```python
from build123d import *

# Parameters (mm, degrees)
BOSS_EXTRUDE1_DEPTH   = 25.4
FILLET1_R             = 6.35
F_8_CLEARANCE_HOLE1_D = 4.4958
F_8_CLEARANCE_HOLE2_D = 4.4958


with BuildPart() as part:
    # Sketch1 → Boss-Extrude1 (new body)
    with BuildSketch(Plane(origin=(0, 0, 0), x_dir=(0, 0, -1), z_dir=(1, 0, 0))):
        Polygon((0, 0), (0, 38.1), (-3.175, 38.1), (-3.175, 3.175), (-38.1, 3.175), (-38.1, 0), align=None)
    extrude(amount=BOSS_EXTRUDE1_DEPTH)

    # Fillet1
    # the kernel refuses this fillet: 6.35 mm, written as the material it adds along each edge
    with BuildSketch(Plane(origin=(0, 3.175, 3.175), x_dir=(0, 1, 0), z_dir=(1, 0, 0))) as fillet1_piece_1:
        with BuildLine():
            CenterArc((FILLET1_R, FILLET1_R), FILLET1_R, 180, 90)
            Line((0, FILLET1_R), (0, 0))
            Line((0, 0), (FILLET1_R, 0))
        make_face()
    extrude(amount=25.4)
    # the kernel refuses this fillet: 6.35 mm, written as the material it takes off along each edge
    with BuildSketch(Plane(origin=(-13.748153285, 38.1, 3.175), x_dir=(0, 0, -1), z_dir=(1, 0, 0))) as fillet1_2_piece_1:
        with BuildLine():
            CenterArc((6.35, -5.499261314), FILLET1_R, 120, 60)
            Line((0, -5.499261314), (0, 0))
            Line((0, 0), (3.175, 0))
        make_face()
    extrude(amount=52.89630657, mode=Mode.SUBTRACT)
    with BuildSketch(Plane(origin=(-13.748153285, 3.175, 38.1), x_dir=(0, -1, 0), z_dir=(1, 0, 0))) as fillet1_2_piece_2:
        with BuildLine():
            CenterArc((6.35, 5.499261314), FILLET1_R, 180, 60)
            Line((0, 5.499261314), (0, 0))
            Line((0, 0), (3.175, 0))
        make_face()
    extrude(amount=52.89630657, mode=Mode.SUBTRACT)

    # #8 Clearance Hole1 (through all)
    with Locations(Plane.XY.offset(3.175)):
        with Locations((12.7, 20.6375)):
            Hole(F_8_CLEARANCE_HOLE1_D / 2)

    # #8 Clearance Hole2 (through all)
    with Locations(Plane(origin=(0, 3.175, 0), x_dir=(1, 0, 0), z_dir=(0, 1, 0))):
        with Locations((12.7, -20.6375)):
            Hole(F_8_CLEARANCE_HOLE2_D / 2)


solid = part.part
```
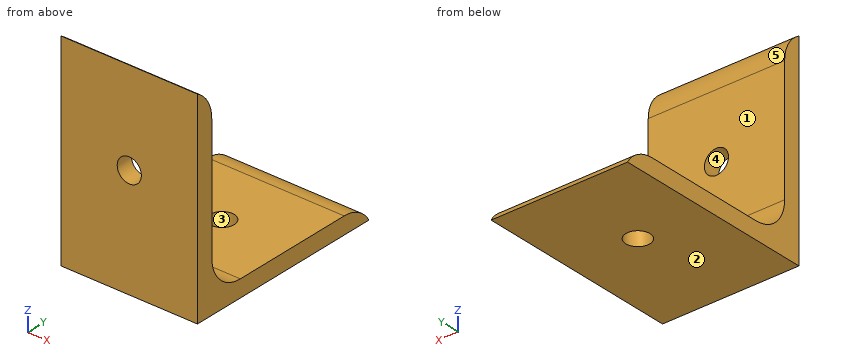
Verification items for the finished model (mm, model axes). Face numbers are marked on the shaded views. A direction names the side the tool comes from. Give positions to 0.01 mm unless a question says otherwise; leave off trailing zeros. Order: outer loops, then holes, each group sorted by start corner. A loop starts at its lowest first (then second) coordinate and runs counter-clockwise, first axis right, second up. Notation, with made-up numbers: M 29.25,11 L 59.25,11 A15 cw 59.25,24 Z; hole C -7.75,0 d6. An arc over 180 degrees is marked long. Return JSON: item names as keys, results as strings. Group by question number.
1) Go/stop test with flat-tipped pins: pin 1 Ø1.5 at (x, y) = (21, 24) entering from -Z; pin 2 Ø3 at (x, y) = (3, 28.5) entering from +Z (3 decimals). Record where each tip stops, or that it passes through.
2) Section check B-B on x = 18.5. Record the cut outline in (y, z) (3 decimals), and give its area (3 significant figures).
3) Scan lines: line 1 (Z direction, x = 10.5, y = 25) (3 decimals); line 2 (Y direction, x = 12.7, z = 0.9). Record each from-to range of solid material in increasing order.
4) Mould release check, pull along Y, two halves, no side actions. Record for the marked faces 3, 4 and 5: pulls with the +Y half, pulls with the -Y half, needs draft (parallel to the pull), parting line crosses it, or undercut.
5) Section check C-C on y = 13.5. Record the cut outline in (x, z) (3 decimals).
6) Section check A-A on x = 12.7. Record the cut outline in (y, z) (3 decimals), and give its area (3 significant figures).
7) Access from +Z, -Z, +X, -X, +Y, -Y to the whole of each face (thin tool, end or side, straight path). Record for the marked faces 1 and 2.
Answer block:
{
 "1": {"pin 1": "stops at z = 0", "pin 2": "stops at z = 3.175"},
 "2": {"outline": "M 0,0 L 38.1,0 A6.35 ccw 32.601,3.175 L 9.525,3.175 A6.35 cw 3.175,9.525 L 3.175,32.601 A6.35 ccw 0,38.1 Z", "area": "230 mm^2"},
 "3": {"line 1": "z = 0 to 3.175", "line 2": "y = 0 to 18.39, 22.89 to 37.47"},
 "4": {"face 3": "undercut", "face 4": "needs draft", "face 5": "pulls with the +Y half"},
 "5": {"outline": "M 0,0 L 25.4,0 L 25.4,3.175 L 0,3.175 Z"},
 "6": {"outline": "M 0,0 L 18.39,0 L 18.39,3.175 L 9.525,3.175 A6.35 cw 3.175,9.525 L 3.175,18.39 L 0,18.39 Z; M 0,22.885 L 3.175,22.885 L 3.175,32.601 A6.35 ccw 0,38.1 Z; M 22.885,0 L 38.1,0 A6.35 ccw 32.601,3.175 L 22.885,3.175 Z", "area": "202 mm^2"},
 "7": {"face 1": "+Z, +X, -X, +Y", "face 2": "-Z, +X, -X, +Y, -Y"}
}
